Input: part model. Units: mm. Frame: model coordinates. Give positions to 0.01 mm unless a question says otherwise; leave off trailing zeros. Write each loop counter-clockwise with the first axis right and the second up, starting at its lowest first coordinate (ties: lowest second). Pieces come first, ordered by that corner, then holes. Notation, with made-up numbers: (32, 21.5) -> (60, 21.5) arc R30 ccw to (60, 51.5) -> close; hole circle Ø9 at (33.25, 19). An arc over 180 degrees is marked (long way). Answer as a JSON object with one key per item and string values. Group by question number.
from build123d import *

# Parameters (mm, degrees)
SKETCH_1_W          = 180
SKETCH_1_H          = 180
EXTRUDE_1_DEPTH     = 10
SKETCH_2_R          = 10
SKETCH_2_R_2        = 3.25
CUT_EXTRUDE_1_DEPTH = 11


with BuildPart() as part:
    # 草图1 → 凸台-拉伸1 (new body)
    with BuildSketch(Plane.XY):
        Rectangle(SKETCH_1_W, SKETCH_1_H)
    extrude(amount=EXTRUDE_1_DEPTH)

    # 草图2 → 切除-拉伸1 (cut)
    with BuildSketch(Plane(origin=(0, 0, 0), x_dir=(-1, 0, 0), z_dir=(0, 0, -1))):
        Circle(SKETCH_2_R)
        with Locations((-22, 0)):
            Circle(SKETCH_2_R_2)
        with Locations((-11, 19.052558883)):
            Circle(SKETCH_2_R_2)
        with Locations((11, 19.052558883)):
            Circle(SKETCH_2_R_2)
        with Locations((22, 0)):
            Circle(SKETCH_2_R_2)
        with Locations((11, -19.052558883)):
            Circle(SKETCH_2_R_2)
        with Locations((-11, -19.052558883)):
            Circle(SKETCH_2_R_2)
        with Locations((65, -20)):
            Circle(SKETCH_2_R_2)
        with Locations((65, -40)):
            Circle(SKETCH_2_R_2)
        with Locations((-65, -20)):
            Circle(SKETCH_2_R_2)
        with Locations((-65, -40)):
            Circle(SKETCH_2_R_2)
    extrude(amount=-CUT_EXTRUDE_1_DEPTH, mode=Mode.SUBTRACT)


solid = part.part
1. Section B-B (y = -40). Return the cut outline in (x, z), plus the area to 3 significant figures.
2. Section D-D (z = 3.5). State how many separate pieces and enclosed holes the cut face has, plus the area to 3 significant figures.
3. Section C-C (y = -6). Return the cut outline in (x, z), plus the area to 3 significant figures.
4. Section A-A (x = -22). Return the cut outline in (y, z), plus the area to 4 significant figures.
5. Line query: line 1 (Y direction, x = -11, z = 7.75); line 2 (Y direction, x = 65, z = 6); line 3 (X direction, y = 0.5, z = 6.5). Output: solid intervals per line, ascending.
6. Mould query, pull axis Y, two halves, no side actions, for faces 1 (the face through (-61.753, -19.857, 4.93)), 2 (the face through (90, -1, 5)), 3 (the face through (-1, -90, 5)). Classes: pulls with the +Y half, pulls with the -Y half, needs draft (parallel to the pull), parting line crosses it, or undercut.
Working result:
{
 "1": {"outline": "(-90, 0) -> (-68.25, 0) -> (-68.25, 10) -> (-90, 10) -> close; (-61.75, 0) -> (61.75, 0) -> (61.75, 10) -> (-61.75, 10) -> close; (68.25, 0) -> (90, 0) -> (90, 10) -> (68.25, 10) -> close", "area": "1,670 mm^2"},
 "2": {"separate pieces": "1", "enclosed holes": "11", "area": "31,800 mm^2"},
 "3": {"outline": "(-90, 0) -> (-8, 0) -> (-8, 10) -> (-90, 10) -> close; (8, 0) -> (90, 0) -> (90, 10) -> (8, 10) -> close", "area": "1,640 mm^2"},
 "4": {"outline": "(-90, 0) -> (-3.25, 0) -> (-3.25, 10) -> (-90, 10) -> close; (3.25, 0) -> (90, 0) -> (90, 10) -> (3.25, 10) -> close", "area": "1,735 mm^2"},
 "5": {"line 1": "y = -90 to -22.3, -15.8 to 15.8, 22.3 to 90", "line 2": "y = -90 to -43.25, -36.75 to -23.25, -16.75 to 90", "line 3": "x = -90 to -25.21, -18.79 to -9.99, 9.99 to 18.79, 25.21 to 90"},
 "6": {"face 1": "undercut", "face 2": "needs draft", "face 3": "pulls with the -Y half"}
}
